The listing builds one solid part. Answer for the finished solid, in the listing's coordinates (mm). Face numbers are marked on the shaded views. A direction names the side the tool comes from. Round coordinates to 2 decimals unless told otherwise and drop trailing zeros. Order: outer loops, then holes, each group sorted by start corner. A loop starts at its lowest first (then second) coordinate and runs counter-clockwise, first axis right, second up. Notation, with made-up numbers: M 3.25,74.25 L 40.25,74.25 A9 ccw 40.25,87.25 Z; hole C -22,49 d5. An arc over 180 degrees is marked long. Put each result on its own line as item: value. Start each with the question number.
1. The part is cut by section B-B (z = 15.75). Give the vertices of the cut face in (x, y).
2. Which of the six approach directions +Z, -Z, +X, -X, +Y, -Y give full straight-line access (tool end or side, diameter ignored) to the marked faces 1, 2 and 3?
3. Each of these flat-tipped pins is pushed along its axis until it touches: pin 1 Ø6 at (x, z) = (51.5, 22.5) entering from +Y; pin 2 Ø4 at (x, z) = (38.5, 13.5) entering from +Y; pin 3 Ø3 at (x, y) = (82, 0.5) entering from -Z. Where does it stop, or does it pass through?
4. The part is cut by section C-C (x = 55). Give the vertices of the cut face in (y, z), then the cut area to 3 significant figures.
5. The part is cut by section A-A (x = 82.5). Give the vertices of the cut face in (y, z), then the cut area to 3 significant figures.
6. Consider line 1 (X direction, y = -2.25, z = 21); line 2 (X direction, y = 1, z = 19.5); line 3 (Z direction, x = 32.5, y = 0). Determine where each line is inside the solid, lowest interval first.
7. The part is cut by section D-D (z = 24). Give the vertices of the cut face in (x, y), then the cut area to 3 significant figures.
from build123d import *

# Parameters (mm, degrees)
F0_W     = 17.018
F0_H     = 3.9243
F6_DEPTH = 6.35


with BuildPart() as f1:
    # F0 (on Front) → F1 (revolve)
    with BuildSketch(Plane.XZ):
        Polygon((25.488018, 25.201135), (14.972418, 25.201135), (14.972418, 17.682735), (25.488018, 17.682735), (25.488018, 23.194535), align=None)
    revolve(axis=Axis((20.230218, 0, 17.682735), (1, 0, 0)))

    # F0 (on Front) → F2 (revolve)
    with BuildSketch(Plane.XZ):
        Polygon((25.488018, 23.194535), (25.488018, 17.682735), (58.152418, 17.682735), (58.152418, 21.670535), (58.152418, 23.194535), align=None)
    revolve(axis=Axis((41.820218, 0, 17.682735), (1, 0, 0)))

    # F0 (on Front) → F3 (revolve)
    with BuildSketch(Plane.XZ):
        Polygon((58.152418, 21.670535), (58.152418, 17.682735), (58.152418, 16.920735), (78.726418, 16.920735), (78.726418, 17.746235), (78.726418, 21.670535), align=None)
    revolve(axis=Axis((68.439418, 0, 16.920735), (1, 0, 0)))

    # F0 (on Front) → F4 (revolve)
    with BuildSketch(Plane.XZ):
        with Locations((87.235418, 19.708385)):
            Rectangle(F0_W, F0_H)
    revolve(axis=Axis((87.235418, 0, 17.746235), (1, 0, 0)))

    # F5 (on face) → F6 (cut)
    with BuildSketch(Plane(origin=(14.972418, 0, 0), x_dir=(0, -1, 0), z_dir=(-1, 0, 0))):
        Polygon((1.436831, 13.369142), (4.454097, 16.770271), (3.017266, 21.083864), (-1.436831, 21.996329), (-4.454097, 18.5952), (-3.017266, 14.281606), align=None)
    extrude(amount=-F6_DEPTH, mode=Mode.SUBTRACT)


solid = f1.part
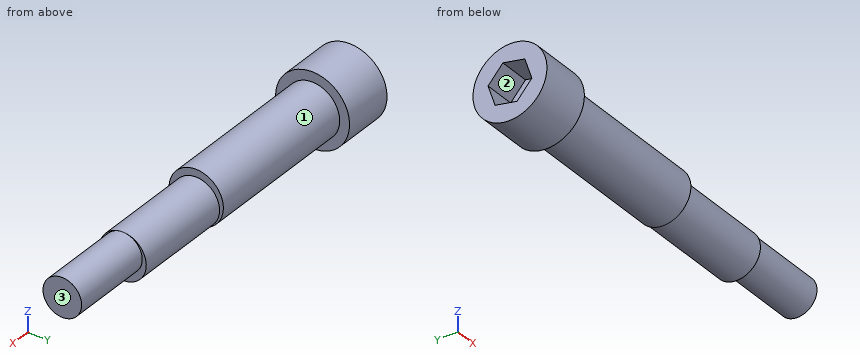
Resolved:
1. outline: M 14.97,-7.27 L 25.49,-7.27 L 25.49,-5.16 L 58.15,-5.16 L 58.15,-4.6 L 78.73,-4.6 L 78.73,-3.38 L 95.74,-3.38 L 95.74,3.38 L 78.73,3.38 L 78.73,4.6 L 58.15,4.6 L 58.15,5.16 L 25.49,5.16 L 25.49,7.27 L 14.97,7.27 L 14.97,3.51 L 21.32,3.51 L 21.32,-3.55 L 14.97,-3.55 Z
2. face 1: +X
2. face 2: -X
2. face 3: +Z, -Z, +X, +Y, -Y
3. pin 1: y = 5.2
3. pin 2: y = 5.06
3. pin 3: z = 13.82
4. outline: C 0,17.68 d11.02
4. area: 95.4 mm2
5. outline: C 0,17.75 d7.85
5. area: 48.4 mm2
6. line 1: 21.32 to 78.73
6. line 2: 21.32 to 95.74
6. line 3: 12.17 to 23.19
7. outline: M 14.97,-4.08 L 25.49,-4.08 L 25.49,4.08 L 14.97,4.08 Z
7. area: 85.7 mm2
